from build123d import *

# Parameters (mm, degrees)
SKETCH_2_W               = 40
SKETCH_2_H               = 40
EXTRUDE_1_DEPTH          = 5
EXTRUDE_2_DEPTH          = 2
HOLE_WIZARD_M5_1_D       = 4.2
HOLE_WIZARD_M5_1_DEPTH   = 12.4
HOLE_WIZARD_M5_1_TIP     = 1.2618073
CUT_EXTRUDE_5_DEPTH      = 74.218850032
CUT_EXTRUDE_5_DEPTH_BACK = 74.218850032
SKETCH_4_R               = 4


with BuildPart() as part:
    # 草图2 → 凸台-拉伸1 (new body)
    with BuildSketch(Plane.XY):
        Rectangle(SKETCH_2_W, SKETCH_2_H)
    extrude(amount=EXTRUDE_1_DEPTH)

    # 草图3 → 凸台-拉伸2 (add)
    with BuildSketch(Plane(origin=(0, 20, 0), x_dir=(1, 0, 0), z_dir=(0, 1, 0))):
        Polygon((20, 0), (20, 55), (-20, 55), (-20, 0), (-20, -5), (20, -5), align=None)
    extrude_2 = extrude(amount=EXTRUDE_2_DEPTH)

    # 镜向1: 凸台-拉伸2 across plane
    add(extrude_2.mirror(Plane.ZX))

    # M5 螺纹孔1
    with Locations(Plane(origin=(-12.5, 12.5, 5), x_dir=(1, 0, 0), z_dir=(0, 0, 1))):
        with Locations((0, 0), (25, 0), (25, -25), (0, -25)):
            Hole(HOLE_WIZARD_M5_1_D / 2, depth=HOLE_WIZARD_M5_1_DEPTH)
            with Locations((0, 0, -(HOLE_WIZARD_M5_1_DEPTH + HOLE_WIZARD_M5_1_TIP / 2))):  # 118° drill point
                Cone(0, HOLE_WIZARD_M5_1_D / 2, HOLE_WIZARD_M5_1_TIP, mode=Mode.SUBTRACT)

    # 草图4 → 切除-拉伸5 (cut, two sides: drawn at the far end of the back side and taken through both)
    with BuildSketch(Plane(origin=(0, -22, 0), x_dir=(1, 0, 0), z_dir=(0, 1, 0)).offset(-CUT_EXTRUDE_5_DEPTH_BACK)):
        with BuildLine():
            Line((13.250714432, 50), (-13.250714432, 50))
            Line((-13.250714432, 50), (-1.167748962, 29.861724217))
            ThreePointArc((-1.167748962, 29.861724217), (0, 30), (1.167748962, 29.861724217))
            Line((1.167748962, 29.861724217), (13.250714432, 50))
        make_face()
        with BuildLine():
            Line((15, 2.915475947), (15, 47.084524053))
            Line((15, 47.084524053), (3.740227739, 28.318236951))
            ThreePointArc((3.740227739, 28.318236951), (4.674459257, 26.774663532), (5, 25))
            ThreePointArc((5, 25), (4.674459257, 23.225336468), (3.740227739, 21.681763049))
            Line((3.740227739, 21.681763049), (15, 2.915475947))
        make_face()
        with BuildLine():
            Line((-3.740227739, 28.318236951), (-15, 47.084524053))
            Line((-15, 47.084524053), (-15, 2.915475947))
            Line((-15, 2.915475947), (-3.740227739, 21.681763049))
            ThreePointArc((-3.740227739, 21.681763049), (-5, 25), (-3.740227739, 28.318236951))
        make_face()
        with BuildLine():
            Line((-1.167748962, 20.138275783), (-13.250714432, 0))
            Line((-13.250714432, 0), (13.250714432, 0))
            Line((13.250714432, 0), (1.167748962, 20.138275783))
            ThreePointArc((1.167748962, 20.138275783), (0, 20), (-1.167748962, 20.138275783))
        make_face()
        with Locations(Location((0, 25, 0), (0, 0, 270))):
            Circle(SKETCH_4_R)
    extrude(amount=CUT_EXTRUDE_5_DEPTH + CUT_EXTRUDE_5_DEPTH_BACK, mode=Mode.SUBTRACT)


solid = part.part
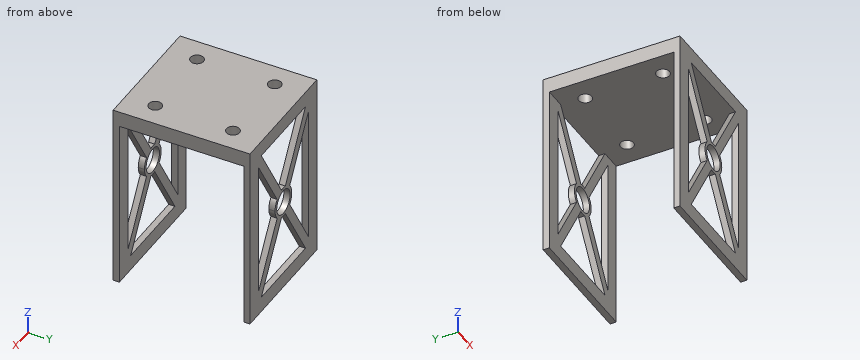
Geometry: final body of the model. Coordinates: model frame, mm. Round coordinates to 2 decimals unless told otherwise and drop trailing zeros. Loops run counter-clockwise (first coordinate to the right, second up) from the corner with the lowest first, then second, coordinate; pieces in that order, holes last.
Q1. Pin query (flat end, axial travel): P1, Ø5, axis at x = 12.5, y = 12.5, coming from the -Z side; P2, Ø3.5, axis at x = 12.5, y = -12.5, coming from the -Z side. Return the tip coordinate at first contact, or that it passes through.
Q2. Material intervals for L1, parallel to Y at x = -12.5, z = 3.65; L2, parallel to X at y = -21, z = -25; L3, parallel to Y at x = -12, z = -5.5, sorted ascending.
Q3. Section D-D on y = 4. Return loops of the section in (x, z), plus the area to 3 significant figures.
Q4. Section A-A on x = 0. Return loops of the section in (y, z).
Q5. Section C-C on z = -4. State how many separate pieces and enclosed holes the cut face has, plus the area to 3 significant figures.
Q6. Section B-B on y = -12.5. Return loops of the section in (x, z).
Evaluation:
1. P1: stops at z = 0
1. P2: passes through
2. L1: y = -22 to -14.6, -10.4 to 10.4, 14.6 to 22
2. L2: x = -20 to -15, -5 to -4, 4 to 5, 15 to 20
2. L3: y = -22 to -20, 20 to 22
3. outline: (-20, 0) - (20, 0) - (20, 5) - (-20, 5) - close
3. area: 200 mm2
4. outline: (-22, -55) - (-20, -55) - (-20, -50) - (-22, -50) - close; (-22, -30) - (-20, -30) - (-20, -29) - (-22, -29) - close; (-22, -21) - (-20, -21) - (-20, -20) - (-22, -20) - close; (-22, 0) - (22, 0) - (22, 5) - (-22, 5) - close; (20, -55) - (22, -55) - (22, -50) - (20, -50) - close; (20, -30) - (22, -30) - (22, -29) - (20, -29) - close; (20, -21) - (22, -21) - (22, -20) - (20, -20) - close
5. separate pieces: 8
5. enclosed holes: 0
5. area: 68.0 mm2
6. outline: (-20, 0) - (-14.6, 0) - (-14.6, 5) - (-20, 5) - close; (-10.4, 0) - (10.4, 0) - (10.4, 5) - (-10.4, 5) - close; (14.6, 0) - (20, 0) - (20, 5) - (14.6, 5) - close
